```python
from build123d import *

# Parameters (mm, degrees)
F0_R     = 11.2
F1_DEPTH = 7


with BuildPart() as f1:
    # F0 (on Top) → F1 (new body)
    with BuildSketch(Plane.XY):
        with BuildLine():
            ThreePointArc((-9.886205, -8.746596), (-13.2, 0), (-9.886205, 8.746596))
            Line((-9.886205, 8.746596), (-17.443001, 8.746596))
            ThreePointArc((-17.443001, 8.746596), (-40.529206, 0), (-17.443001, -8.746596))
            Line((-17.443001, -8.746596), (-9.886205, -8.746596))
        make_face()
        with Locations((-27.329206, 0)):
            Circle(F0_R, mode=Mode.SUBTRACT)
        with BuildLine():
            ThreePointArc((9.886205, 8.746596), (12.343782, 4.676649), (13.2, 0))
            ThreePointArc((13.2, 0), (12.343782, -4.676649), (9.886205, -8.746596))
            Line((9.886205, -8.746596), (17.443001, -8.746596))
            ThreePointArc((17.443001, -8.746596), (40.529206, 0), (17.443001, 8.746596))
            Line((17.443001, 8.746596), (9.886205, 8.746596))
        make_face()
        with Locations((27.329206, 0)):
            Circle(F0_R, mode=Mode.SUBTRACT)
        with BuildLine():
            ThreePointArc((9.886205, -8.746596), (12.343782, -4.676649), (13.2, 0))
            ThreePointArc((13.2, 0), (12.343782, 4.676649), (9.886205, 8.746596))
            ThreePointArc((9.886205, 8.746596), (0, 13.2), (-9.886205, 8.746596))
            ThreePointArc((-9.886205, 8.746596), (-13.2, 0), (-9.886205, -8.746596))
            ThreePointArc((-9.886205, -8.746596), (0, -13.2), (9.886205, -8.746596))
        make_face()
        Circle(F0_R, mode=Mode.SUBTRACT)
    extrude(amount=F1_DEPTH)


solid = f1.part
```
The listing builds one solid part. Answer for the finished solid, in the listing's coordinates (mm). A direction names the side the tool comes from. Round coordinates to 2 decimals unless told otherwise and drop trailing zeros. Loops run counter-clockwise (first coordinate to the right, second up) from the corner with the lowest first, then second, coordinate; pieces in that order, holes last.
Q1. Which of the six approach directions +Z, -Z, +X, -X, +Y, -Y give full straight-line access (tool end or side, diameter ignored) to faces 1 (the face through (14, -8.747, 3)), 2 (the face through (40.52, -0.45, 3.45)), 3 (the face through (-14, 8.747, 3))?
Q2. Section D-D, the plane y = 3.75 is taken. Determine the outline of the cut face in (x, z), then the cut area to 3 significant figures.
Q3. Given pin 1 Ø2 at (x, z) = (-14, 2.5) entering from -Y; pin 2 Ø3 at (y, z) = (-3.5, 1.5) entering from -X; pin 3 Ø2 at (x, z) = (-13.5, 5.5) entering from +Y; pin 4 Ø12 at (x, y) = (-6.5, -6.5) entering from -Z, each flat-ended and moving along its own axis, determine where each tip first touches the part or whether it passes through.
Q4. Section A-A, the plane y = 0 is taken. Determine the outline of the cut face in (x, z).
Q5. Section B-B, the plane x = 0 is taken. Determine the outline of the cut face in (y, z), then the cut area to 3 significant figures.
Q6. Find the intervals of material crossed by line 1 (X direction, y = -7.75, z = 5.75); line 2 (X direction, y = 5.5, z = 1.5); line 3 (Y direction, x = 27.5, z = 0.75), in increasing order.
Q7. Section C-C, the plane z = 5 is taken. Determine the outline of the cut face in (x, y).
Completed:
1. face 1: +Z, -Z, -Y
1. face 2: +Z, -Z
1. face 3: +Z, -Z, +Y
2. outline: (-39.99, 0) - (-37.88, 0) - (-37.88, 7) - (-39.99, 7) - close; (-16.78, 0) - (-10.55, 0) - (-10.55, 7) - (-16.78, 7) - close; (10.55, 0) - (16.78, 0) - (16.78, 7) - (10.55, 7) - close; (37.88, 0) - (39.99, 0) - (39.99, 7) - (37.88, 7) - close
2. area: 117 mm2
3. pin 1: stops at y = -8.75
3. pin 2: stops at x = -40.38
3. pin 3: stops at y = 8.75
3. pin 4: stops at z = 0
4. outline: (-40.53, 0) - (-38.53, 0) - (-38.53, 7) - (-40.53, 7) - close; (-16.13, 0) - (-11.2, 0) - (-11.2, 7) - (-16.13, 7) - close; (11.2, 0) - (16.13, 0) - (16.13, 7) - (11.2, 7) - close; (38.53, 0) - (40.53, 0) - (40.53, 7) - (38.53, 7) - close
5. outline: (-13.2, 0) - (-11.2, 0) - (-11.2, 7) - (-13.2, 7) - close; (11.2, 0) - (13.2, 0) - (13.2, 7) - (11.2, 7) - close
5. area: 28.0 mm2
6. line 1: x = -38.01 to -35.41, -19.24 to -8.09, 8.09 to 19.24, 35.41 to 38.01
6. line 2: x = -39.33 to -37.09, -17.57 to -9.76, 9.76 to 17.57, 37.09 to 39.33
6. line 3: y = -13.2 to -11.2, 11.2 to 13.2
7. outline: (-17.44, -8.75) - (-9.89, -8.75) arc R13.2 ccw to (9.89, -8.75) - (17.44, -8.75) arc R13.2 ccw (long way) to (17.44, 8.75) - (9.89, 8.75) arc R13.2 ccw to (-9.89, 8.75) - (-17.44, 8.75) arc R13.2 ccw (long way) to start; hole circle Ø22.4 at (-27.33, 0); hole circle Ø22.4 at (0, 0); hole circle Ø22.4 at (27.33, 0)
